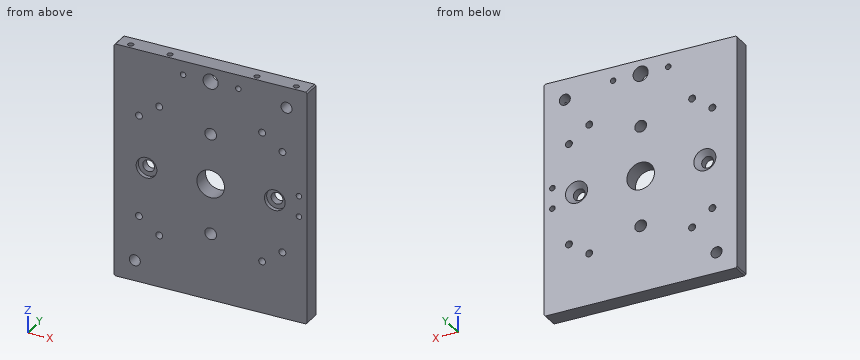
```python
from build123d import *

# Parameters (mm, degrees)
F0_W           = 140
F0_H           = 170
F1_DEPTH       = 12
F2_R           = 10
F3_DEPTH       = 12
F5_D           = 8
F6_R           = 7.5
F7_DEPTH       = 3
F9_D           = 8.5
F9_DEPTH       = 12
F9_CSINK_D     = 16
F9_CSINK_ANGLE = 90
F9_TIP         = 2.5536576309
F11_D          = 8.5
F13_D          = 5
F15_D          = 4
F16_R          = 5.5
F17_DEPTH      = 12
F19_D          = 4
F19_DEPTH      = 13
F19_TIP        = 1.2017212381
F20_SIZE       = 1


with BuildPart() as f1:
    # F0 (on Front) → F1 (new body)
    with BuildSketch(Plane.XZ):
        Rectangle(F0_W, F0_H)
    extrude(amount=F1_DEPTH)

    # F2 (on face) → F3 (cut)
    with BuildSketch(Plane.XZ.offset(12)):
        Circle(F2_R)
    extrude(amount=-F3_DEPTH, mode=Mode.SUBTRACT)

    # F5 (through all)
    with Locations(Plane.XZ.offset(12)):
        with Locations((-55, -70), (55, 70)):
            Hole(F5_D / 2)

    # F6 (on face) → F7 (cut)
    with BuildSketch(Plane.XZ.offset(12)):
        with Locations((-46.5, 0)):
            Circle(F6_R)
        with Locations((46.5, 0)):
            Circle(F6_R)
    extrude(amount=-F7_DEPTH, mode=Mode.SUBTRACT)

    # F9
    with Locations(Plane(origin=(0, 0, 0), x_dir=(-1, 0, 0), z_dir=(0, 1, 0))):
        with Locations((46.5, 0), (-46.5, 0)):
            CounterSinkHole(F9_D / 2, F9_CSINK_D / 2, depth=F9_DEPTH, counter_sink_angle=F9_CSINK_ANGLE)
            with Locations((0, 0, -(F9_DEPTH + F9_TIP / 2))):  # 118° drill point
                Cone(0, F9_D / 2, F9_TIP, mode=Mode.SUBTRACT)

    # F11 (through all)
    with Locations(Plane.XZ.offset(12)):
        with Locations((0, -36.5), (0, 36.5)):
            Hole(F11_D / 2)

    # F13 (through all)
    with Locations(Plane.XZ.offset(12)):
        with Locations((52, -36.8), (37.3, -47.2), (-37.3, -47.2), (-52, -36.8), (-52, 36.8), (-37.3, 47.2), (37.3, 47.2), (52, 36.8)):
            Hole(F13_D / 2)

    # F15 (through all)
    with Locations(Plane.XZ.offset(12)):
        with Locations((-20, 75), (20, 75), (64, 7.5), (64, -7.5)):
            Hole(F15_D / 2)

    # F16 (on face) → F17 (cut)
    with BuildSketch(Plane.XZ.offset(12)):
        with Locations((0, 75)):
            Circle(F16_R)
    extrude(amount=-F17_DEPTH, mode=Mode.SUBTRACT)

    # F19
    with Locations(Plane.XY.offset(85)):
        with Locations((60, -8), (31.5, -8), (-31.5, -8), (-60, -8)):
            Hole(F19_D / 2, depth=F19_DEPTH)
            with Locations((0, 0, -(F19_DEPTH + F19_TIP / 2))):  # 118° drill point
                Cone(0, F19_D / 2, F19_TIP, mode=Mode.SUBTRACT)

    # F20
    f20_edges = [f1.edges().sort_by_distance(p)[0] for p in [
        (-70, -6, -85),
        (-70, -6, 85),
        (70, -6, 85),
        (70, -6, -85),
    ]]
    chamfer(f20_edges, length=F20_SIZE)


solid = f1.part
```
Build history of the part. All positions in model axes, mm. Give positions to 0.01 mm unless a question says otherwise; leave off trailing zeros. Order: outer loops, then holes, each group sorted by start corner. A loop starts at its lowest first (then second) coordinate and runs counter-clockwise, first axis right, second up. Notation, with made-up numbers: M 65,-39.5 L 94,-39.5 A8 cw 94,-34.5 Z; hole C 33.25,23 d8. An arc over 180 degrees is marked long. Write item = value, one per line. Start each with the question number.
(1) Slice it at B-B on x = 64. Write the cut outline in (y, z).
(2) Pin check, flat tips, straight feed: pin 1 Ø11 at (x, z) = (-46.5, 0) entering from -Y; pin 2 Ø13.5 at (x, z) = (46.5, 0) entering from +Y. Stop position of each tip, or through.
(3) Probe L1, parallel to Z at x = 64, y = -6.5; L2, parallel to X at y = -9.25, z = 47.5; L3, parallel to Z at x = 0.5, y = -5.5. List the from-to ranges inside material, lowest first. Write a range as [from, to].
(4) Slice it at A-A on z = 47.2. Write the cut outline in (x, y), plus the area to 3 significant figures.
Responses:
q1.outline = M -12,-85 L 0,-85 L 0,-9.5 L -12,-9.5 Z; M -12,-5.5 L 0,-5.5 L 0,5.5 L -12,5.5 Z; M -12,9.5 L 0,9.5 L 0,85 L -12,85 Z
q2.pin_1 = -9
q2.pin_2 = -1.25
q3.L1 = [-85, -9.5], [-5.5, 5.5], [9.5, 85]
q3.L2 = [-70, -39.78], [-34.82, 34.82], [39.78, 70]
q3.L3 = [-85, -40.72], [-32.28, -9.99], [9.99, 32.28], [40.72, 69.52], [80.48, 85]
q4.outline = M -70,-12 L -39.8,-12 L -39.8,0 L -70,0 Z; M -34.8,-12 L 34.8,-12 L 34.8,0 L -34.8,0 Z; M 39.8,-12 L 70,-12 L 70,0 L 39.8,0 Z
q4.area = 1,560 mm2
